Could you check a few things on this model? Use its own coordinates, in mm. Face numbers are marked on the shaded views. Give positions to 0.01 mm unless a question says otherwise; leave off trailing zeros. Order: outer loops, then holes, each group sorted by start corner. A loop starts at its lowest first (then second) coordinate and runs counter-clockwise, first axis right, second up. Notation, with made-up numbers: (74, 82.25) -> (92, 82.25) arc R12 ccw to (92, 102.25) -> close; hole circle Ø6 at (56.5, 15). An arc over 180 degrees is marked (long way). Write each question's results on one line, items separated by ' | '.
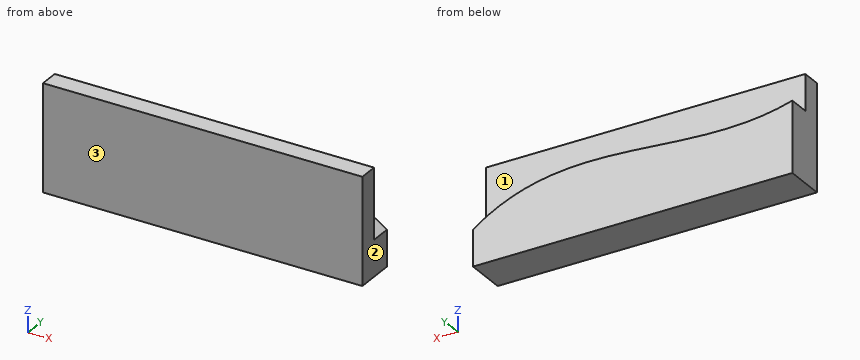
```python
from build123d import *

# Parameters (mm, degrees)
SKETCH1_W           = 150
SKETCH1_H           = 50
BOSS_EXTRUDE1_DEPTH = 19
CUT_EXTRUDE1_DEPTH  = 10


with BuildPart() as part:
    # Sketch1 → Boss-Extrude1 (new body)
    with BuildSketch(Plane(origin=(0, 0, 0), x_dir=(1, 0, 0), z_dir=(0, 1, 0))):
        with Locations((75, 25)):
            Rectangle(SKETCH1_W, SKETCH1_H)
    extrude(amount=BOSS_EXTRUDE1_DEPTH)

    # Sketch2 → Cut-Extrude1 (cut)
    with BuildSketch(Plane(origin=(0, 19, 0), x_dir=(1, 0, 0), z_dir=(0, 1, 0))):
        with BuildLine():
            Line((-14.15766915, 11.43597738), (-14.15766915, -14.105632465))
            Line((-14.15766915, -14.105632465), (161.61937252, -14.105632465))
            Line((161.61937252, -14.105632465), (161.61937252, 43.164685263))
            add(Edge.make_bspline(
                [(-14.15766915, 11.43597738), (43.406827576, 39.699894181), (110.750368018, -9.289380037), (161.61937252, 43.164685263)],
                knots=[0, 0, 0, 0, 1, 1, 1, 1], degree=3))
        make_face()
    extrude(amount=-CUT_EXTRUDE1_DEPTH, mode=Mode.SUBTRACT)


solid = part.part
```
Q1. I need wall thicknesses on line 1 along Y through (x, z) = (67, -7.5); line 2 along X through (y, z) = (13.5, -32.5); line 3 along Z through (x, y) = (8.5, 13.5). Which ranges of each line are inside material? Lowest first, please.
Here are the results:
line 1: y = 0 to 9 | line 2: x = 0 to 149.2 | line 3: z = -50 to -18.89
Q2. Suppose I cut it at A-A on z = -8. Please give me the cut outline in (x, y).
Here are the results:
outline: (0, 0) -> (150, 0) -> (150, 9) -> (0, 9) -> close
Q3. Thinking about a two-plate mould opening in Y: for the marked faces 1, 2 and 3, which applies, +Y half, -Y half, draft (parallel to the pull), parting line (faces both ways), or undercut?
Here are the results:
face 1: +Y half | face 2: draft | face 3: -Y half
